Geometry: final body of the model. Coordinates: model frame, mm. A direction names the side the tool comes from. Give positions to 0.01 mm unless a question says otherwise; leave off trailing zeros. Order: outer loops, then holes, each group sorted by start corner. A loop starts at its lowest first (then second) coordinate and runs counter-clockwise, first axis right, second up. Notation, with made-up numbers: (17, 19.5) -> (27, 19.5) arc R7 ccw to (27, 23.5) -> close; hole circle Ø11 at (-21, -32.75). An arc over 180 degrees is marked (long way). Write item = value, one per line.
```python
from build123d import *

# Parameters (mm, degrees)
CROQUIS1_R              = 50
SALIENTE_EXTRUIR1_DEPTH = 3
CORTAR_EXTRUIR1_REACH   = 5
CROQUIS2_R              = 1.5
CORTAR_EXTRUIR2_REACH   = 5
CROQUIS3_W              = 6
CROQUIS3_H              = 60


with BuildPart() as part:
    # Croquis1 → Saliente-Extruir1 (new body)
    with BuildSketch(Plane(origin=(0, 0, 0), x_dir=(1, 0, 0), z_dir=(0, 1, 0))):
        Circle(CROQUIS1_R)
    extrude(amount=SALIENTE_EXTRUIR1_DEPTH)

    # Croquis2 → Cortar-Extruir1 (cut, up to next)
    with BuildSketch(Plane(origin=(0, 3, 0), x_dir=(1, 0, 0), z_dir=(0, 1, 0)), mode=Mode.PRIVATE) as cortar_extruir1_sk1:
        with Locations((0, 6)):
            Circle(CROQUIS2_R)
    cortar_extruir1_tool1 = extrude(cortar_extruir1_sk1.sketch, amount=-CORTAR_EXTRUIR1_REACH, mode=Mode.PRIVATE) & part.part
    add(cortar_extruir1_tool1.solids().sort_by_distance((0, 3, -6))[0], mode=Mode.SUBTRACT)
    # Croquis2 → Cortar-Extruir1 (cut, up to next)
    with BuildSketch(Plane(origin=(0, 3, 0), x_dir=(1, 0, 0), z_dir=(0, 1, 0)), mode=Mode.PRIVATE) as cortar_extruir1_sk2:
        with Locations((6, 0)):
            Circle(CROQUIS2_R)
    cortar_extruir1_tool2 = extrude(cortar_extruir1_sk2.sketch, amount=-CORTAR_EXTRUIR1_REACH, mode=Mode.PRIVATE) & part.part
    add(cortar_extruir1_tool2.solids().sort_by_distance((6, 3, 0))[0], mode=Mode.SUBTRACT)
    # Croquis2 → Cortar-Extruir1 (cut, up to next)
    with BuildSketch(Plane(origin=(0, 3, 0), x_dir=(1, 0, 0), z_dir=(0, 1, 0)), mode=Mode.PRIVATE) as cortar_extruir1_sk3:
        with Locations((0, -6)):
            Circle(CROQUIS2_R)
    cortar_extruir1_tool3 = extrude(cortar_extruir1_sk3.sketch, amount=-CORTAR_EXTRUIR1_REACH, mode=Mode.PRIVATE) & part.part
    add(cortar_extruir1_tool3.solids().sort_by_distance((0, 3, 6))[0], mode=Mode.SUBTRACT)
    # Croquis2 → Cortar-Extruir1 (cut, up to next)
    with BuildSketch(Plane(origin=(0, 3, 0), x_dir=(1, 0, 0), z_dir=(0, 1, 0)), mode=Mode.PRIVATE) as cortar_extruir1_sk4:
        with Locations((-6, 0)):
            Circle(CROQUIS2_R)
    cortar_extruir1_tool4 = extrude(cortar_extruir1_sk4.sketch, amount=-CORTAR_EXTRUIR1_REACH, mode=Mode.PRIVATE) & part.part
    add(cortar_extruir1_tool4.solids().sort_by_distance((-6, 3, 0))[0], mode=Mode.SUBTRACT)

    # Croquis3 → Cortar-Extruir2 (cut, up to next)
    with BuildSketch(Plane(origin=(0, 3, 0), x_dir=(1, 0, 0), z_dir=(0, 1, 0)), mode=Mode.PRIVATE) as cortar_extruir2_sk1:
        with Locations((22, 0)):
            Rectangle(CROQUIS3_W, CROQUIS3_H)
    cortar_extruir2_tool1 = extrude(cortar_extruir2_sk1.sketch, amount=-CORTAR_EXTRUIR2_REACH, mode=Mode.PRIVATE) & part.part
    add(cortar_extruir2_tool1.solids().sort_by_distance((22, 3, 0))[0], mode=Mode.SUBTRACT)
    # Croquis3 → Cortar-Extruir2 (cut, up to next)
    with BuildSketch(Plane(origin=(0, 3, 0), x_dir=(1, 0, 0), z_dir=(0, 1, 0)), mode=Mode.PRIVATE) as cortar_extruir2_sk2:
        with Locations((-22, 0)):
            Rectangle(CROQUIS3_W, CROQUIS3_H)
    cortar_extruir2_tool2 = extrude(cortar_extruir2_sk2.sketch, amount=-CORTAR_EXTRUIR2_REACH, mode=Mode.PRIVATE) & part.part
    add(cortar_extruir2_tool2.solids().sort_by_distance((-22, 3, 0))[0], mode=Mode.SUBTRACT)


solid = part.part
```
1) First-contact query: P1, Ø0.9, axis at y = 1, z = -6, coming from the -X side; P2, Ø0.9, axis at y = 1, z = -5.5, coming from the +X side; P3, Ø1.5, axis at y = 1, z = 8, coming from the +X side. Flat tips, straight axial feed; report the tip coordinate or a pass-through.
Check sheet entries:
P1 = -49.69
P2 = 49.74
P3 = 49.47
2) Mould query, pull axis X, two halves, no side actions, for faces 1 (the face through (47.69, 1.48, -15.02)), 2 (the face through (-1, 3, -1)), 3 (the face through (-0.325, 1.521, -4.536)). Classes: +X half, -X half, draft (parallel to the pull), parting line (faces both ways), or undercut.
Check sheet entries:
face_1 = parting line
face_2 = draft
face_3 = undercut
3) Line query: line 1 (Z direction, x = 0, y = 1.4); line 2 (X direction, y = 0.8, z = 0); line 3 (X direction, y = 2, z = 6). Output: solid intervals per line, ascending. Write a range as from..to.
Check sheet entries:
line_1 = -50..-7.5, -4.5..4.5, 7.5..50
line_2 = -50..-25, -19..-7.5, -4.5..4.5, 7.5..19, 25..50
line_3 = -49.64..-25, -19..-1.5, 1.5..19, 25..49.64
4) Section query D-D (z = -16.5). Output: boundary loops of the cut face in (x, y), plus the area to 3 significant figures.
Check sheet entries:
outline = (-47.2, 0) -> (-25, 0) -> (-25, 3) -> (-47.2, 3) -> close; (-19, 0) -> (19, 0) -> (19, 3) -> (-19, 3) -> close; (25, 0) -> (47.2, 0) -> (47.2, 3) -> (25, 3) -> close
area = 247 mm²
5) Section query A-A (y = 1.55). Output: boundary loops of the cut face in (x, z), plus the area to 3 significant figures.
Check sheet entries:
outline = circle Ø100 at (0, 0); hole (-25, -30) -> (-19, -30) -> (-19, 30) -> (-25, 30) -> close; hole circle Ø3 at (-6, 0); hole circle Ø3 at (0, -6); hole circle Ø3 at (0, 6); hole circle Ø3 at (6, 0); hole (19, -30) -> (25, -30) -> (25, 30) -> (19, 30) -> close
area = 7,110 mm²
6) Section query C-C (x = 0). Output: boundary loops of the cut face in (y, z), plus the area to 3 significant figures.
Check sheet entries:
outline = (0, -50) -> (3, -50) -> (3, -7.5) -> (0, -7.5) -> close; (0, -4.5) -> (3, -4.5) -> (3, 4.5) -> (0, 4.5) -> close; (0, 7.5) -> (3, 7.5) -> (3, 50) -> (0, 50) -> close
area = 282 mm²
7) Reachability of faces 4 (the face through (-1, 0, -1)), 5 (the face through (19, 2, 0)) from +Z, -Z, +X, -X, +Y, -Y: full face, straight path, thin tool, end or side. Return the list, or none.
Check sheet entries:
face_4 = +Z, -Z, +X, -X, -Y
face_5 = +Y, -Y
8) Section query B-B (z = 0). Output: boundary loops of the cut face in (x, y).
Check sheet entries:
outline = (-50, 0) -> (-25, 0) -> (-25, 3) -> (-50, 3) -> close; (-19, 0) -> (-7.5, 0) -> (-7.5, 3) -> (-19, 3) -> close; (-4.5, 0) -> (4.5, 0) -> (4.5, 3) -> (-4.5, 3) -> close; (7.5, 0) -> (19, 0) -> (19, 3) -> (7.5, 3) -> close; (25, 0) -> (50, 0) -> (50, 3) -> (25, 3) -> close
